from build123d import *

# Parameters (mm, degrees)
CROQUIS1_R                   = 25
SALIENTE_EXTRUIR1_DEPTH      = 20
SALIENTE_EXTRUIR2_DEPTH      = 40
SALIENTE_EXTRUIR2_DEPTH_BACK = 1
CROQUIS2_R                   = 15
CROQUIS3_R                   = 10
CORTAR_EXTRUIR1_DEPTH        = 40


with BuildPart() as part:
    # Croquis1 → Saliente-Extruir1 (new body)
    with BuildSketch(Plane.XY):
        with Locations(Location((0, 0, 0), (0, 0, 180))):
            Circle(CROQUIS1_R)
    extrude(amount=SALIENTE_EXTRUIR1_DEPTH)

    # Croquis2 → Saliente-Extruir2 (add, two sides: drawn at the far end of the back side and taken through both)
    with BuildSketch(Plane.XY.offset(20).offset(-SALIENTE_EXTRUIR2_DEPTH_BACK)):
        Circle(CROQUIS2_R)
    extrude(amount=SALIENTE_EXTRUIR2_DEPTH + SALIENTE_EXTRUIR2_DEPTH_BACK)

    # Croquis3 → Cortar-Extruir1 (cut)
    with BuildSketch(Plane.XY.offset(60)):
        Circle(CROQUIS3_R)
    extrude(amount=-CORTAR_EXTRUIR1_DEPTH, mode=Mode.SUBTRACT)


solid = part.part
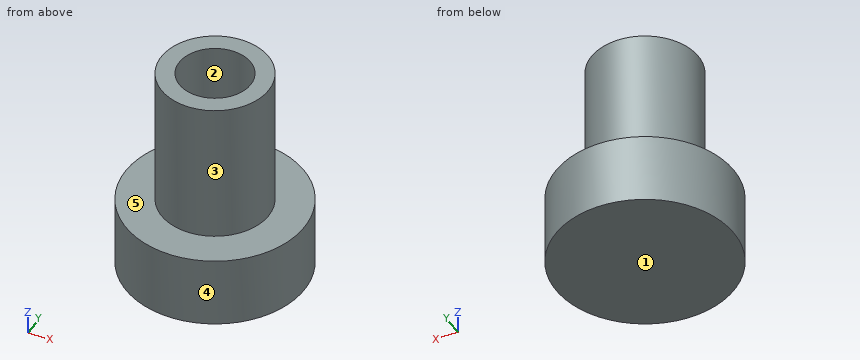
Source: CAD feature listing. Evaluate the final solid. Frame: model axes, mm. Face numbers are marked on the shaded views. A direction names the side the tool comes from. Give positions to 0.01 mm unless a question says otherwise; leave off trailing zeros. Write each loop counter-clockwise with the first axis right and the second up, starting at its lowest first coordinate (ties: lowest second). Pieces come first, ordered by that corner, then holes. Notation, with made-up numbers: M 48,-12.5 L 64,-12.5 A30 cw 64,9.5 Z; hole C -33,-29.5 d4. An arc over 180 degrees is marked long. Return JSON: item names as keys, results as strings. Group by question number.
1) Set-up query: the marked faces 4 and 5. Return all of +Z, -Z, +X, -X, +Y, -Y with unobstructed straight access to the full face (end or side cutting, diameter ignored); none if empty.
2) Cut plane A-A, the plane x = 0. Output: boundary loops of the cut face in (y, z), then the cut area to 3 significant figures.
3) Cut plane D-D, the plane z = 5. Output: boundary loops of the cut face in (x, y).
4) Cut plane B-B, the plane y = -6. Output: boundary loops of the cut face in (x, z).
5) Cut plane C-C, the plane z = 23.5. Output: boundary loops of the cut face in (x, y), then the cut area to 3 significant figures.
6) Draft query along Y for the marked faces 1, 2 and 3. Return one class per face: released by +Y, released by -Y, zero draft, split by the parting line, or undercut.
7) Ray query, L1, parallel to Y at x = 0, z = 34; L2, parallel to Z at x = 5, y = -7.5; L3, parallel to Y at x = -6.5, z = 53. Return the intervals inside material, ascending.
8) First-contact query: pin 1 Ø6 at (y, z) = (-7.5, 9) entering from -X; pin 2 Ø16 at (x, y) = (1, -0.5) entering from +Z; pin 3 Ø1 at (x, y) = (-10.5, -15.5) entering from -Z; pin 4 Ø8 at (y, z) = (7.5, 45) entering from -X. Flat tips, straight axial feed; report the tip coordinate or a pass-through.
Data:
{
 "1": {"face 4": "+Z, -Z", "face 5": "+Z"},
 "2": {"outline": "M -25,0 L 25,0 L 25,20 L 15,20 L 15,60 L 10,60 L 10,20 L -10,20 L -10,60 L -15,60 L -15,20 L -25,20 Z", "area": "1,400 mm²"},
 "3": {"outline": "C 0,0 d50"},
 "4": {"outline": "M -24.27,0 L 24.27,0 L 24.27,20 L 13.75,20 L 13.75,60 L 8,60 L 8,20 L -8,20 L -8,60 L -13.75,60 L -13.75,20 L -24.27,20 Z"},
 "5": {"outline": "C 0,0 d30; hole C 0,0 d20", "area": "393 mm²"},
 "6": {"face 1": "zero draft", "face 2": "undercut", "face 3": "split by the parting line"},
 "7": {"L1": "y = -15 to -10, 10 to 15", "L2": "z = 0 to 20", "L3": "y = -13.52 to -7.6, 7.6 to 13.52"},
 "8": {"pin 1": "stops at x = -24.59", "pin 2": "stops at z = 20", "pin 3": "stops at z = 0", "pin 4": "stops at x = -14.59"}
}
